from build123d import *

# Parameters (mm, degrees)
BOSS_EXTRUDE1_DEPTH = 45
SKETCH2_R           = 25
SKETCH2_R_2         = 30
BOSS_EXTRUDE2_DEPTH = 35
CUT_EXTRUDE1_DEPTH  = 10


with BuildPart() as part:
    # Sketch1 → Boss-Extrude1 (new, symmetric)
    with BuildSketch(Plane.XY):
        with BuildLine():
            Line((-50, 212.5), (-74.416342412, -178.161478599))
            ThreePointArc((-74.416342412, -178.161478599), (0, -262.5), (74.416342412, -178.161478599))
            Line((74.416342412, -178.161478599), (50, 212.5))
            ThreePointArc((50, 212.5), (0, 262.5), (-50, 212.5))
        make_face()
    extrude(amount=BOSS_EXTRUDE1_DEPTH, both=True)

    # Sketch2 → Boss-Extrude2 (add)
    with BuildSketch(Plane.XY.offset(45)):
        with Locations((0, 212.5)):
            Circle(SKETCH2_R)
        with Locations((0, -187.5)):
            Circle(SKETCH2_R_2)
    boss_extrude2 = extrude(amount=BOSS_EXTRUDE2_DEPTH)

    # Mirror1: Boss-Extrude2 across plane
    add(boss_extrude2.mirror(Plane.XY))

    # Sketch3 → Cut-Extrude1 (cut)
    with BuildSketch(Plane.XY.offset(45)):
        with BuildLine():
            Line((15, 96.352828314), (15, -96.352828314))
            ThreePointArc((15, -96.352828314), (0, -111.352828314), (-15, -96.352828314))
            Line((-15, -96.352828314), (-15, 96.352828314))
            ThreePointArc((-15, 96.352828314), (0, 111.352828314), (15, 96.352828314))
        make_face()
    cut_extrude1 = extrude(amount=-CUT_EXTRUDE1_DEPTH, mode=Mode.SUBTRACT)

    # Mirror2: Cut-Extrude1 across plane
    add(cut_extrude1.mirror(Plane.XY), mode=Mode.SUBTRACT)


solid = part.part
Work out the finished part from the listing and answer in its coordinate system (mm). A direction names the side the tool comes from. Round coordinates to 2 decimals unless told otherwise and drop trailing zeros. Write each loop counter-clockwise with the first axis right and the second up, starting at its lowest first coordinate (ties: lowest second). Pieces come first, ordered by that corner, then holes.
1) A cutting plane is placed at D-D (y = 101). Give the vertices of the cut face in (x, z), plus the area to 3 significant figures.
2) A cutting plane is placed at C-C (x = 0). Give the vertices of the cut face in (y, z).
3) Given pin 1 Ø8 at (y, z) = (8, 41) entering from +X; pin 2 Ø6 at (y, z) = (60, 34.5) entering from -X; pin 3 Ø24 at (x, y) = (-5.5, -13) entering from -Z, each flat-ended and moving along its own axis, determine where each tip first touches the part or whether it passes through.
4) A cutting plane is placed at B-B (z = -57). Give the vertices of the cut face in (x, y), plus the area to 3 significant figures.
5) A cutting plane is placed at A-A (y = -187.5). Give the vertices of the cut face in (x, z).
6) The mould has two halves that part along X. Classify faces 1 (the flat face through (-62.037, 19.904, 0.63)), 2 (the flat face through (0, 213, -80)), 3 (the cylindrical face through (0.33, -111.35, 40.07)): pulls with the +X half, pulls with the -X half, needs draft (parallel to the pull), parting line crosses it, or undercut.
7) Straight lines are drawn through the part: line 1 (Y direction, x = 1, z = -70); line 2 (Z direction, x = -44.5, y = -220); line 3 (Z direction, x = 11, y = -8). For each, find the intervals that lie inside material, in ascending order.
8) A tool of negligible diameter and unlimited length cuts with its end or side. For faces 4 (the cylindrical face through (-3.255, 237.287, -62.255)), 5 (the flat face through (0, 2, 35)), 6 (the flat face through (0, 213, 80)), from which of +Z, -Z, +X, -X, +Y, -Y can it reach the whole face along a straight path? Write none if from no direction.
Completed:
1. outline: (-56.97, -45) - (-14.26, -45) - (-14.26, -35) - (14.26, -35) - (14.26, -45) - (56.97, -45) - (56.97, 45) - (14.26, 45) - (14.26, 35) - (-14.26, 35) - (-14.26, 45) - (-56.97, 45) - close
1. area: 9,680 mm2
2. outline: (-262.5, -45) - (-217.5, -45) - (-217.5, -80) - (-157.5, -80) - (-157.5, -45) - (-111.35, -45) - (-111.35, -35) - (111.35, -35) - (111.35, -45) - (187.5, -45) - (187.5, -80) - (237.5, -80) - (237.5, -45) - (262.5, -45) - (262.5, 45) - (237.5, 45) - (237.5, 80) - (187.5, 80) - (187.5, 45) - (111.35, 45) - (111.35, 35) - (-111.35, 35) - (-111.35, 45) - (-157.5, 45) - (-157.5, 80) - (-217.5, 80) - (-217.5, 45) - (-262.5, 45) - close
3. pin 1: stops at x = 63.03
3. pin 2: stops at x = -59.72
3. pin 3: stops at z = -45
4. outline: circle Ø60 at (0, -187.5); circle Ø50 at (0, 212.5)
4. area: 4,790 mm2
5. outline: (-75, -45) - (-30, -45) - (-30, -80) - (30, -80) - (30, -45) - (75, -45) - (75, 45) - (30, 45) - (30, 80) - (-30, 80) - (-30, 45) - (-75, 45) - close
6. face 1: pulls with the -X half
6. face 2: needs draft
6. face 3: undercut
7. line 1: y = -217.48 to -157.52, 187.52 to 237.48
7. line 2: z = -45 to 45
7. line 3: z = -35 to 35
8. face 4: -Z
8. face 5: +Z
8. face 6: +Z, +X, -X, +Y, -Y
